Autodesk Inventor part; units mm, degrees
ref_plane "YZ Plane" through (0, 0, 0) normal (1, 0, 0) x (0, 1, 0)
ref_plane "XZ Plane" through (0, 0, 0) normal (0, 1, 0) x (-1, 0, 0)
ref_plane "XY Plane" through (0, 0, 0) normal (0, 0, 1) x (1, 0, 0)
sketch "草图1" plane through (0, 0, 0) normal (1, 0, 0) x (0, 1, 0)
  circle A0 centre (0, 0) radius 33.5
  circle A1 centre (33.5, 0) radius 5
  circle A2 centre (-16.75, 29.0119) radius 5
  circle A3 centre (-16.75, -29.0119) radius 5
  line L0 (33.5, 5) -> (18.5, 5)
  line L1 (18.5, 5) -> (18.5, -5)
  line L2 (18.5, -5) -> (33.5, -5)
  line L3 (33.5, -5) -> (33.5, 5)
  line L4 (-21.0801, 26.5119) -> (-13.5801, 13.5215)
  line L5 (-4.9199, 18.5215) -> (-12.4199, 31.5119)
  line L6 (-12.4199, -31.5119) -> (-4.9199, -18.5215)
  line L7 (-13.5801, -13.5215) -> (-21.0801, -26.5119)
  arc A4 (-4.9199, 18.5215) -> (18.5, 5) centre (18.5, 32.0429) ccw
  circle A5 centre (22.5, 0) radius 1.5
  line L8 (26.5, 5) -> (26.5, -5)
  arc A6 (-13.5801, -13.5215) -> (-13.5801, 13.5215) centre (-37, 0) ccw
  line L9 (-17.5801, 20.4497) -> (-8.9199, 25.4497)
  circle A7 centre (-11.25, 19.4856) radius 1.5
  arc A8 (18.5, -5) -> (-4.9199, -18.5215) centre (18.5, -32.0429) ccw
  line L10 (-8.9199, -25.4497) -> (-17.5801, -20.4497)
  circle A9 centre (-11.25, -19.4856) radius 1.5
  circle A10 centre (0, 0) radius 5
  point P0 (-4.9199, -18.5215)
  point P1 (18.5, -5)
  point P2 (-8.9199, 25.4497)
  point P3 (-13.5801, 13.5215)
  point P4 (-13.5801, -13.5215)
  point P5 (-17.5801, -20.4497)
  point P6 (-8.9199, -25.4497)
  dimension "d0" = 67
  dimension "d1" = 10
  dimension "d6" = 360
  dimension "d8" = 15
  dimension "d11" = 360
  dimension "d13" = 3
  dimension "d14" = 11
  dimension "d15" = 7
  dimension "d18" = 360
  dimension "d20" = 10
extrude "拉伸1" add sketch "草图1" along normal blind 3 contours L8 L2 L1 L0 | L5 A4 L1 A8 L6 L10 L7 A6 L4 L9
equation "\"折弯半径\" = 厚度"
equation "\"折弯释压宽度\" = 厚度"
equation "\"折弯释压深度\" = 0.5 * 厚度"
equation "\"拐角释压尺寸\" = 4 * 厚度"
equation "\"最小余量\" = 2 * 厚度"
equation "\"过渡半径\" = 折弯半径"
equation "\"Jacobi半径尺寸\" = 折弯半径"
equation "\"间隙大小\" = 厚度"
properties part number "CAR_TRI_FRAME"
Source: CAD feature listing. Evaluate the final solid. Frame: model axes, mm. A direction names the side the tool comes from. Coordinates: 2 decimals unless noted, no trailing zeros. Loops run counter-clockwise (first coordinate to the right, second up) from the corner with the lowest first, then second, coordinate; pieces in that order, holes last. Notation, with made-up numbers: (-12, 17) - (0, 17) arc R18 cw to (0, 52) - close; hole circle Ø8 at (-8, 85). An arc over 180 degrees is marked (long way). One line per question, with ' | ' between items.
1) Section A-A, the plane y = 22.5. Return loops of the section in (x, z).
Report:
outline: (0, -5) - (3, -5) - (3, -1.5) - (0, -1.5) - close; (0, 1.5) - (3, 1.5) - (3, 5) - (0, 5) - close
2) Section C-C, the plane x = 1.35. Return loops of the section in (y, z), then the cut area to 3 significant figures.
Report:
outline: (-17.58, -20.45) - (-8.92, -25.45) - (-4.92, -18.52) arc R27.04 cw to (18.5, -5) - (26.5, -5) - (26.5, 5) - (18.5, 5) arc R27.04 cw to (-4.92, 18.52) - (-8.92, 25.45) - (-17.58, 20.45) - (-13.58, 13.52) arc R27.04 cw to (-13.58, -13.52) - close; hole circle Ø3 at (-11.25, -19.49); hole circle Ø3 at (-11.25, 19.49); hole circle Ø10 at (0, 0); hole circle Ø3 at (22.5, 0) | area: 770 mm²
3) Pull-direction query (Y, two-part tool) for faces 1 (the face through (1.479, -13.311, 22.915)), 2 (the face through (1, 26.5, 0)), 3 (the face through (1.48, -11.58, 20.95)); classes: released by +Y, released by -Y, zero draft, split by the parting line, or undercut.
Report:
face 1: released by -Y | face 2: released by +Y | face 3: undercut
4) Line query: line 1 along Z through (x, y) = (0.7, 22.5); line 2 along Y through (x, z) = (1.85, -1); line 3 along Y through (x, z) = (1.65, 19.5). Output: solid intervals per line, ascending.
Report:
line 1: z = -5 to -1.5, 1.5 to 5 | line 2: y = -9.98 to -4.9, 4.9 to 21.38, 23.62 to 26.5 | line 3: y = -17.03 to -12.75, -9.75 to -5.48
5) Set-up query: faces 4 (the face through (1.479, -11.575, -18.021)), 5 (the face through (1, 22, -5)), 6 (the face through (1.479, -13.189, -22.985)), 7 (the face through (1.479, -15.608, 17.034)), 8 (the face through (1, 23, 5)). Return all of +Z, -Z, +X, -X, +Y, -Y with unobstructed straight access to the full face (end or side cutting, diameter ignored); none if empty.
Report:
face 4: +X, -X | face 5: -Z, +X, -X, +Y | face 6: -Z, +X, -X, -Y | face 7: +X, -X, -Y | face 8: +Z, +X, -X, +Y
6) First-contact query: P1, Ø1.5, axis at x = 2, y = 24, coming from the -Z side; P2, Ø2.5, axis at y = -11.25, z = 19.49, coming from the +X side; P3, Ø1.5, axis at x = 1.5, y = 22, coming from the +Z side; P4, Ø1, axis at x = 2, y = -9.5, coming from the -Z side. Flat tips, straight axial feed; report the tip coordinate or a pass-through.
Report:
P1: stops at z = -5 | P2: passes through | P3: stops at z = 5 | P4: stops at z = -25.4
7) Section B-B, the plane z = 0. Return loops of the section in (x, y), then the cut area to 3 significant figures.
Report:
outline: (0, -9.96) - (3, -9.96) - (3, -5) - (0, -5) - close; (0, 5) - (3, 5) - (3, 21) - (0, 21) - close; (0, 24) - (3, 24) - (3, 26.5) - (0, 26.5) - close | area: 70.4 mm²
8) Section D-D, the plane y = -11.25. Return loops of the section in (x, z), then the cut area to 3 significant figures.
Report:
outline: (0, -24.1) - (3, -24.1) - (3, -20.99) - (0, -20.99) - close; (0, -17.99) - (3, -17.99) - (3, -8.26) - (0, -8.26) - close; (0, 8.26) - (3, 8.26) - (3, 17.99) - (0, 17.99) - close; (0, 20.99) - (3, 20.99) - (3, 24.1) - (0, 24.1) - close | area: 77.1 mm²
